from build123d import *

# Parameters (mm, degrees)
SKETCH1_W           = 94
SKETCH1_H           = 83
SKETCH1_R           = 1.5875
BOSS_EXTRUDE1_DEPTH = 2
SKETCH2_R           = 1.1
CUT_EXTRUDE1_DEPTH  = 10
SKETCH3_W           = 42
SKETCH3_H           = 24
CUT_EXTRUDE2_DEPTH  = 0.2


with BuildPart() as part:
    # Sketch1 → Boss-Extrude1 (new body)
    with BuildSketch(Plane(origin=(0, 0, 0), x_dir=(1, 0, 0), z_dir=(0, 1, 0))):
        Rectangle(SKETCH1_W, SKETCH1_H)
        with Locations((-42, 36.5)):
            Circle(SKETCH1_R, mode=Mode.SUBTRACT)
        with Locations((42, 36.5)):
            Circle(SKETCH1_R, mode=Mode.SUBTRACT)
        with Locations((42, -36.5)):
            Circle(SKETCH1_R, mode=Mode.SUBTRACT)
        with Locations((-42, -36.5)):
            Circle(SKETCH1_R, mode=Mode.SUBTRACT)
    extrude(amount=BOSS_EXTRUDE1_DEPTH)

    # Sketch2 → Cut-Extrude1 (cut)
    with BuildSketch(Plane(origin=(0, 2, 0), x_dir=(1, 0, 0), z_dir=(0, 1, 0))):
        with Locations((-39.5, 9.75)):
            Circle(SKETCH2_R)
        with Locations((-1.5, 9.75)):
            Circle(SKETCH2_R)
        with Locations((-1.5, -9.75)):
            Circle(SKETCH2_R)
        with Locations((-39.5, -9.75)):
            Circle(SKETCH2_R)
        with BuildLine():
            Line((40.172144385, 2), (47, 2))
            Line((47, 2), (47, -2))
            Line((47, -2), (40.172144385, -2))
            ThreePointArc((40.172144385, -2), (33.25, 0), (40.172144385, 2))
        make_face()
        Polygon((-18.415, -41.5), (-15.875, -38.96), (15.875, -38.96), (18.415, -41.5), align=None)
        Polygon((-18.415, 41.5), (-15.875, 38.96), (15.875, 38.96), (18.415, 41.5), align=None)
    extrude(amount=-CUT_EXTRUDE1_DEPTH, mode=Mode.SUBTRACT)

    # Sketch3 → Cut-Extrude2 (cut)
    with BuildSketch(Plane(origin=(0, 2, 0), x_dir=(1, 0, 0), z_dir=(0, 1, 0))):
        with Locations((-20.5, 0)):
            Rectangle(SKETCH3_W, SKETCH3_H)
    extrude(amount=-CUT_EXTRUDE2_DEPTH, mode=Mode.SUBTRACT)


solid = part.part
Geometry: final body of the model. Coordinates: model frame, mm. A direction names the side the tool comes from. Give positions to 0.01 mm unless a question says otherwise; leave off trailing zeros. Write each loop counter-clockwise with the first axis right and the second up, starting at its lowest first coordinate (ties: lowest second). Pieces come first, ordered by that corner, then holes. Notation, with made-up numbers: (-35, -13) - (21, -13) arc R13 cw to (21, -3) - close; hole circle Ø9 at (9, 33.25). An arc over 180 degrees is marked (long way). Return JSON: item names as keys, results as strings. Group by question number.
1) Section D-D on x = -13. Return the cut outline in (y, z).
2) First-contact query: P1, Ø7, axis at x = -26, z = 1.5, coming from the +Y side; P2, Ø1, axis at x = 4, y = 1.5, coming from the -Z side. Flat tips, straight axial feed; report the tip coordinate or a pass-through.
3) Section B-B on y = 1.1. State how many separate pieces and enclosed holes the cut face has, plus the area to 3 significant figures.
4) Section C-C on z = -5. Return the cut outline in (x, y), plus the area to 3 significant figures.
5) Line query: line 1 (X direction, y = 0.4, z = -9.75); line 2 (Z direction, x = -39.5, y = 0.8); line 3 (Z direction, x = -1.5, y = 1.15). Output: solid intervals per line, ascending.
6) Set-up query: faces 1 (the flat face through (44, 1, 2)), 2 (the flat face through (-21, 1.8, 0)), 3 (the flat face through (17.127, 1.014, 40.212)), 4 (the flat face through (-47, 1, 1)), 5 (the cylindrical face through (-1.738, 0.913, -8.676)). Return all of +Z, -Z, +X, -X, +Y, -Y with unobstructed straight access to the full face (end or side cutting, diameter ignored); none if empty.
7) Mould query, pull axis Z, two halves, no side actions, for faces 6 (the cylindrical face through (43.514, 0.986, -36.977)), 7 (the flat face through (-33, 1, 41.5)), 8 (the cylindrical face through (-40.486, 0.986, 36.023)), 9 (the flat face through (-17.163, 1.014, -40.248)). Classes: released by +Z, released by -Z, zero draft, split by the parting line, or undercut.
8) Section A-A on x = 37. Return the cut outline in (y, z), plus the area to 3 significant figures.
Filled in:
{
 "1": {"outline": "(0, -38.96) - (2, -38.96) - (2, -12) - (1.8, -12) - (1.8, 12) - (2, 12) - (2, 38.96) - (0, 38.96) - close"},
 "2": {"P1": "stops at y = 1.8", "P2": "stops at z = -38.96"},
 "3": {"separate pieces": "1", "enclosed holes": "8", "area": "7,510 mm^2"},
 "4": {"outline": "(-47, 0) - (47, 0) - (47, 2) - (0.5, 2) - (0.5, 1.8) - (-41.5, 1.8) - (-41.5, 2) - (-47, 2) - close", "area": "180 mm^2"},
 "5": {"line 1": "x = -47 to -40.6, -38.4 to -2.6, -0.4 to 47", "line 2": "z = -41.5 to -10.85, -8.65 to 8.65, 10.85 to 41.5", "line 3": "z = -38.96 to -10.85, -8.65 to 8.65, 10.85 to 38.96"},
 "6": {"face 1": "+X, +Y, -Y", "face 2": "+Y", "face 3": "+Z, +Y, -Y", "face 4": "+Z, -Z, -X, +Y, -Y", "face 5": "+Y, -Y"},
 "7": {"face 6": "undercut", "face 7": "released by +Z", "face 8": "undercut", "face 9": "released by -Z"},
 "8": {"outline": "(0, -41.5) - (2, -41.5) - (2, -3.75) - (0, -3.75) - close; (0, 3.75) - (2, 3.75) - (2, 41.5) - (0, 41.5) - close", "area": "151 mm^2"}
}
